Input: part model. Units: mm. Frame: model coordinates. A direction names the side the tool comes from. Coordinates: 2 decimals unless noted, no trailing zeros. Loops run counter-clockwise (first coordinate to the right, second up) from the corner with the lowest first, then second, coordinate; pieces in that order, holes last. Notation, with made-up numbers: (42, 86.25) -> (66, 86.25) arc R10 cw to (66, 98.25) -> close; hole circle Ø4 at (-2.75, -28). An arc over 180 degrees is marked (long way). Put each result on its own line as item: value. Start each with the question number.
1) Cut plane D-D (x = -8). Return the cut outline in (y, z).
2) Cut plane B-B (y = -18). Return the cut outline in (x, z).
3) Cut plane A-A (x = 0). Return the cut outline in (y, z).
4) Pull-direction query (Y, two-part tool) for faces 1 (the flat face through (-6, -18, -35)), 2 (the flat face through (11.01, -12.14, -19.72)), 3 (the flat face through (0, -19.15, -67)); classes: pulls with the +Y half, pulls with the -Y half, needs draft (parallel to the pull), parting line crosses it, or undercut.
5) Contact query for flat-ended pins moving along their axis: P1, Ø10, axis at x = 7.5, z = -21.5, coming from the +Y side; P2, Ø0.7, axis at y = -18, z = -68.5, coming from the +X side; P3, Ø1.8, axis at y = -18.5, z = -67.5, coming from the -X side. Output: stop coordinate, or through.
6) Cut plane C-C (z = -14). Return the cut outline in (x, y) (1 decimal).
7) Set-up query: faces 4 (the flat face through (-4.65, -18, -67)), 5 (the flat face through (6, -18, -35)), 6 (the flat face through (-11.01, -12.14, -19.72)). Return all of +Z, -Z, +X, -X, +Y, -Y with unobstructed straight access to the full face (end or side cutting, diameter ignored); none if empty.
8) Material intervals for L1, parallel to Y at x = 0, z = 1.95; L2, parallel to Z at x = 8, y = 6; L3, parallel to Z at x = 7, y = -16, sorted ascending.
Autodesk Inventor part; units mm, degrees
ref_plane "YZ Plane" through (0, 0, 0) normal (1, 0, 0) x (0, 1, 0)
ref_plane "XZ Plane" through (0, 0, 0) normal (0, 1, 0) x (-1, 0, 0)
ref_plane "XY Plane" through (0, 0, 0) normal (0, 0, 1) x (1, 0, 0)
sketch "Sketch1" plane through (0, 0, 0) normal (0, 0, 1) x (1, 0, 0)
  circle A0 centre (0, 0) radius 5.15
  circle A1 centre (0, 0) radius 16
  line L0 (-16, 0) -> (-16, -20)
  line L1 (-16, -20) -> (16, -20)
  line L2 (16, -20) -> (16, 0)
  circle A2 centre (0, 0) radius 14.5
  point P0 (-8, 0)
  point P1 (8, 0)
  dimension "d0" = 10.3
  dimension "d1" = 32
  dimension "d3" = 20
  dimension "d4" = 8
  dimension "d5" = 8
  dimension "d28" = 1.5
extrude "Extrusion1" add sketch "Sketch1" along normal blind 3 contours A1 | L2 L1 L0 A1 | A2
hole "Hole1" at (-8, 0, 0) at (8, 0, 0) direction (0, 0, 1) diameter 2.3 end through all
sketch "Sketch2" plane through (0, 0, 0) normal (0, 0, -1) x (-1, 0, 0)
  arc A0 (1.3828, 14.685) -> (-1.3828, 14.685) centre (0, 0) ccw
  line L0 (-1.3828, 14.685) -> (-1.5, 15.9295)
  arc A1 (16, 0) -> (-16, 0) centre (0, 0) ccw
  line L1 (1.3828, 14.685) -> (1.5, 15.9295)
  point P0 (0, 14.75)
  dimension "d15" = 3
  dimension "d16" = 1.25
extrude "Extrusion2" add sketch "Sketch2" along normal blind 15
sketch "Sketch3" plane through (0, 0, 0) normal (0, 0, -1) x (-1, 0, 0)
  arc A0 (-1.9403, 14.7378) -> (1.9403, 14.7378) centre (0, 0) ccw
  arc A1 (-2.3319, 17.7122) -> (2.3319, 17.7122) centre (0, 0) ccw
  line L0 (-6, -16.8273) -> (-6, -20)
  line L1 (-6, -20) -> (6, -20)
  line L2 (16, -20) -> (-16, -20) construction
  line L3 (6, -16.8273) -> (6, -20)
  line L4 (-12, -13.2347) -> (-9.9849, -11.0123)
  line L5 (12, -13.2347) -> (9.9849, -11.0123)
  point P0 (0, 0)
  dimension "d19" = 3
  dimension "d20" = 12
  dimension "d21" = 24
  dimension "d22" = 12
extrude "Extrusion3" add sketch "Sketch3" along normal blind 40
chamfer "Chamfer1" distance 0.5 angle 45 2 edges at (-8, -1.15, 3) (8, -1.15, 3)
sketch "Sketch4" plane through (0, 0, -40) normal (0, 0, -1) x (-1, 0, 0)
  line L0 (-6, -20) -> (6, -20)
  line L1 (6, -20) -> (6, -16.8273)
  line L2 (6, -20) -> (6, -16)
  line L3 (6, -16) -> (-6, -16)
  line L4 (-6, -16.8273) -> (-6, -20)
  line L5 (-6, -16) -> (-6, -20)
  point P0 (0, 0)
  dimension "d29" = 4
extrude "Extrusion4" add sketch "Sketch4" along normal blind 30
sketch "Sketch6" plane through (0, 0, -70) normal (0, 0, -1) x (-1, 0, 0)
  line L0 (-4.65, -16.85) -> (4.65, -16.85)
  line L1 (4.65, -16.85) -> (4.65, -19.15)
  line L2 (4.65, -19.15) -> (-4.65, -19.15)
  line L3 (-4.65, -19.15) -> (-4.65, -16.85)
  line L4 (-6, -20) -> (6, -20)
  line L5 (6, -20) -> (6, -16)
  point P0 (0, 0)
  point P1 (0, -16.85)
  point P2 (0, -20)
  point P3 (4.65, -18)
  point P4 (6, -18)
  dimension "d36" = 2.3
  dimension "d37" = 9.3
extrude "Extrusion5" cut sketch "Sketch6" against normal blind 6
properties part number "Motor Face Mount"
Results found:
1. outline: (-20, 0) -> (-15.97, 0) -> (-15.97, -40) -> (-12.53, -40) -> (-12.53, 0) -> (-1.15, 0) -> (-1.15, 2.5) -> (-1.65, 3) -> (-20, 3) -> close; (1.15, 0) -> (13.86, 0) -> (13.86, 3) -> (1.65, 3) -> (1.15, 2.5) -> close
2. outline: (-16, 0) -> (-6, 0) -> (-6, -70) -> (-4.65, -70) -> (-4.65, -64) -> (4.65, -64) -> (4.65, -70) -> (6, -70) -> (6, 0) -> (16, 0) -> (16, 3) -> (-16, 3) -> close
3. outline: (-20, -70) -> (-19.15, -70) -> (-19.15, -64) -> (-16.85, -64) -> (-16.85, -70) -> (-16, -70) -> (-16, -40) -> (-14.86, -40) -> (-14.86, 0) -> (-5.15, 0) -> (-5.15, 3) -> (-20, 3) -> close; (5.15, 0) -> (14.75, 0) -> (14.75, -15) -> (16, -15) -> (16, 3) -> (5.15, 3) -> close
4. face 1: needs draft
4. face 2: pulls with the +Y half
4. face 3: undercut
5. P1: stops at y = -11.01
5. P2: stops at x = 6
5. P3: stops at x = -6
6. outline: (-12, -13.2) arc R17.9 ccw to (-6, -16.8) -> (-6, -20) -> (6, -20) -> (6, -16.8) arc R17.9 ccw to (12, -13.2) -> (10, -11) arc R14.9 cw to (-10, -11) -> close; (-1.5, 15.9) -> (-1.4, 14.7) arc R14.7 cw to (1.4, 14.7) -> (1.5, 15.9) arc R16 ccw to start
7. face 4: -Z
7. face 5: -Z, +X, -Y
7. face 6: -Z, -X, +Y
8. L1: y = -20 to -5.15, 5.15 to 16
8. L2: z = 0 to 3
8. L3: z = -40 to 3
